Check sheet for the modelled part. Datum: model origin and axes. Units: mm. Face numbers are marked on the shaded views. A direction names the side the tool comes from. Round coordinates to 2 decimals unless told otherwise and drop trailing zeros. Loops run counter-clockwise (first coordinate to the right, second up) from the corner with the lowest first, then second, coordinate; pieces in that order, holes last. Notation, with made-up numbers: (3.5, 81) -> (25.5, 81) arc R31 cw to (25.5, 105) -> close; hole circle Ø8 at (52.25, 71.5). An arc over 180 degrees is marked (long way). Use one line per item in the form item = value. Start each with the question number.
(1) Go/stop test with flat-tipped pins: pin 1 (4 mm diameter, centred on x = 24.39, y = 24.39, fed in from +Z); pin 2 (11 mm diameter, centred on x = 4, y = -0.5, fed in from +Z); pin 3 (3 mm diameter, centred on x = -6.5, z = 2, fed in from -Y); pin 4 (4 mm diameter, centred on x = 15.5, y = 11, fed in from +Z). Record where each tip stops, or that it passes through.
(2) Set-up check for the marked faces 1 and 2: record each of +Z, -Z, +X, -X, +Y, -Y from which the full face is reachable in a straight line by a thin tool's end or side.
(3) Material ranges on probe 1 along Y at (x, z) = (0, 12); probe 2 along X at (y, z) = (23.5, 2.25); probe 3 along X at (y, z) = (6, 7), recorded low to high. Write a range as [from, to].
(4) Sectioned sample at B-B (z = 2.5). Record the cut outline in (x, y).
(5) Sectioned sample at C-C (x = 0). Record the cut outline in (y, z), and give its area (3 significant figures).
(6) Sectioned sample at D-D (y = 0). Record the cut outline in (x, z), and give its area (3 significant figures).
(7) Draft check along X on the marked faces 3, 4 and 5. Enter one of: released by +X, released by -X, zero draft, split by the parting line, or undercut.
(8) Sectioned sample at A-A (y = 24.39). Record the cut outline in (x, z).
from build123d import *

# Parameters (mm, degrees)
BOSS_EXTRUDE1_DEPTH      = 3.81
BOSS_EXTRUDE2_START      = -3.81
SKETCH2_R                = 8.5344
SKETCH2_R_2              = 6.6294
BOSS_EXTRUDE2_DEPTH      = 17.4752
SKETCH4_R                = 6.6294
CUT_EXTRUDE2_DEPTH       = 4.81
SKETCH5_R                = 11.0744
SKETCH5_R_2              = 8.5344
BOSS_EXTRUDE3_DEPTH      = 1.27
BOSS_EXTRUDE3_DEPTH_BACK = 3.81
F_8_CLEARANCE_HOLE1_D    = 4.4958


with BuildPart() as part:
    # Sketch1 → Boss-Extrude1 (new body)
    with BuildSketch(Plane.XY):
        with BuildLine():
            Line((-24.39, 32.01), (24.39, 32.01))
            ThreePointArc((24.39, 32.01), (31.257886274, 27.690990477), (30.340348343, 19.629983761))
            Line((30.340348343, 19.629983761), (8.925522514, -7.140024359))
            ThreePointArc((8.925522514, -7.140024359), (0, -11.43), (-8.925522514, -7.140024359))
            Line((-8.925522514, -7.140024359), (-30.340348343, 19.629983761))
            ThreePointArc((-30.340348343, 19.629983761), (-31.257886274, 27.690990477), (-24.39, 32.01))
        make_face()
    extrude(amount=BOSS_EXTRUDE1_DEPTH)

    # Sketch2 → Boss-Extrude2 (add)
    with BuildSketch(Plane.XY.offset(3.81).offset(BOSS_EXTRUDE2_START)):
        Circle(SKETCH2_R)
        Circle(SKETCH2_R_2, mode=Mode.SUBTRACT)
    extrude(amount=BOSS_EXTRUDE2_DEPTH)

    # Sketch4 → Cut-Extrude2 (cut, through all)
    with BuildSketch(Plane.XY.offset(3.81)):
        Circle(SKETCH4_R)
    extrude(amount=-CUT_EXTRUDE2_DEPTH, mode=Mode.SUBTRACT)

    # Sketch5 → Boss-Extrude3 (add, two sides)
    with BuildSketch(Plane.XY.offset(3.81)) as boss_extrude3_sk:
        Circle(SKETCH5_R)
        Circle(SKETCH5_R_2, mode=Mode.SUBTRACT)
    extrude(amount=BOSS_EXTRUDE3_DEPTH)
    extrude(boss_extrude3_sk.sketch, amount=-BOSS_EXTRUDE3_DEPTH_BACK)

    # #8 Clearance Hole1 (through all)
    with Locations(Plane.XY.offset(3.81)):
        with Locations((-24.39, 24.39), (24.39, 24.39)):
            Hole(F_8_CLEARANCE_HOLE1_D / 2)


solid = part.part
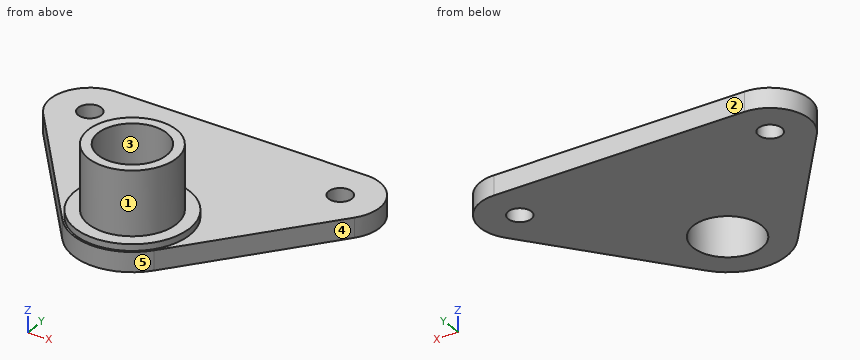
Checks:
q1.pin_1 = through
q1.pin_2 = 17.48
q1.pin_3 = -10.28
q1.pin_4 = 3.81
q2.face_1 = +Z
q2.face_2 = +Z, -Z, +X, -X, +Y
q3.probe_1 = [-8.53, -6.63], [6.63, 8.53]
q3.probe_2 = [-31.96, -26.45], [-22.33, 22.33], [26.45, 31.96]
q3.probe_3 = [-6.07, -2.82], [2.82, 6.07]
q4.outline = (-30.34, 19.63) -> (-8.93, -7.14) arc R11.43 ccw to (8.93, -7.14) -> (30.34, 19.63) arc R7.62 ccw to (24.39, 32.01) -> (-24.39, 32.01) arc R7.62 ccw to start; hole circle Ø4.5 at (-24.39, 24.39); hole circle Ø13.26 at (0, 0); hole circle Ø4.5 at (24.39, 24.39)
q5.outline = (-11.43, 0) -> (-6.63, 0) -> (-6.63, 17.48) -> (-8.53, 17.48) -> (-8.53, 5.08) -> (-11.07, 5.08) -> (-11.07, 3.81) -> (-11.43, 3.81) -> close; (6.63, 0) -> (32.01, 0) -> (32.01, 3.81) -> (11.07, 3.81) -> (11.07, 5.08) -> (8.53, 5.08) -> (8.53, 17.48) -> (6.63, 17.48) -> close
q5.area = 174 mm2
q6.outline = (-14.64, 0) -> (-6.63, 0) -> (-6.63, 17.48) -> (-8.53, 17.48) -> (-8.53, 5.08) -> (-11.07, 5.08) -> (-11.07, 3.81) -> (-14.64, 3.81) -> close; (6.63, 0) -> (14.64, 0) -> (14.64, 3.81) -> (11.07, 3.81) -> (11.07, 5.08) -> (8.53, 5.08) -> (8.53, 17.48) -> (6.63, 17.48) -> close
q6.area = 120 mm2
q7.face_3 = undercut
q7.face_4 = released by +X
q7.face_5 = split by the parting line
q8.outline = (-32.01, 0) -> (-26.64, 0) -> (-26.64, 3.81) -> (-32.01, 3.81) -> close; (-22.14, 0) -> (22.14, 0) -> (22.14, 3.81) -> (-22.14, 3.81) -> close; (26.64, 0) -> (32.01, 0) -> (32.01, 3.81) -> (26.64, 3.81) -> close
